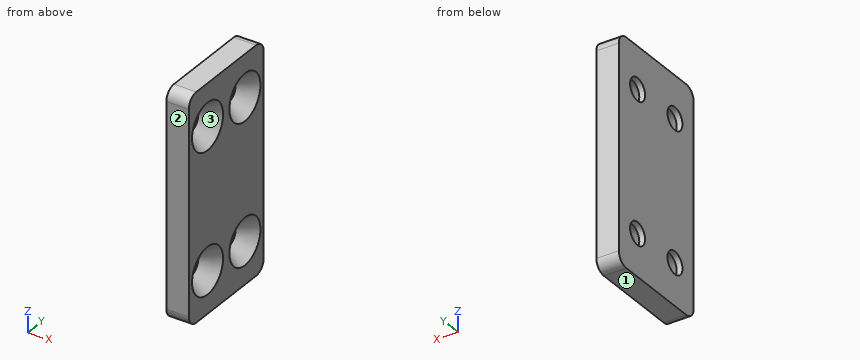
Autodesk Inventor part; units mm, degrees
ref_plane "YZ Plane" through (0, 0, 0) normal (1, 0, 0) x (0, 1, 0)
ref_plane "XZ Plane" through (0, 0, 0) normal (0, 1, 0) x (-1, 0, 0)
ref_plane "XY Plane" through (0, 0, 0) normal (0, 0, 1) x (1, 0, 0)
sketch "Leg_Base_Skt" plane through (0, 0, 0) normal (1, 0, 0) x (0, 1, 0)
  line L0 (-10, -20) -> (10, -20)
  line L1 (10, -20) -> (10, 20)
  line L2 (10, 20) -> (-10, 20)
  line L3 (-10, 20) -> (-10, -20)
  line L4 (-10, -20) -> (10, 20) construction
  line L5 (10, -20) -> (-10, 20) construction
  point P0 (0, 0)
  dimension "d0" = 20
  dimension "d1" = 40
extrude "Leg_Base" add sketch "Leg_Base_Skt" along normal blind 4
sketch "Hole_Base_Skt" plane through (4, 0, 0) normal (1, 0, 0) x (0, 0, -1)
  line L0 (-5, -10) -> (-5, 10) construction
  line L1 (20, 10) -> (-20, 10)
  line L2 (-12.5, 0) -> (-12.5, 10) construction
  line L3 (-12.5, 0) -> (-12.5, -10) construction
  line L4 (-20, -10) -> (20, -10) construction
  line L5 (5, -10) -> (5, 10) construction
  line L6 (20, -10) -> (20, 10) construction
  line L7 (5, 0) -> (20, 0) construction
  line L8 (12.5, 0) -> (12.5, 10) construction
  line L9 (12.5, 0) -> (12.5, -10) construction
  line L10 (-20, 10) -> (-20, -10)
  line L11 (-20, 0) -> (-5, 0) construction
  point P0 (0, 0)
  point P1 (-12.5, -5)
  point P2 (-12.5, 5)
  point P3 (12.5, -5)
  point P4 (12.5, 5)
  dimension "d7" = 15
  dimension "d8" = 15
hole "Hole_Base" at (4, -5, 12.5) at (4, 5, 12.5) at (4, -5, -12.5) at (4, 5, -12.5) direction (-1, 0, 0) diameter 4 end through all countersink diameter 8.3 countersink angle 71.667
fillet "Fillet" radius 2 4 edges at (2, -10, 20) (2, 10, 20) (2, -10, -20) (2, 10, -20)
equation "\"d0\" = block_width"
equation "\"d1\" = ceramic_width + block_height + wood_width"
equation "\"d2\" = screw_head_height + screw_tolerance"
equation "\"d7\" = wood_width"
equation "\"d8\" = block_height"
equation "\"d28\" = screw_body_diam + screw_tolerance"
equation "\"d32\" = screw_head_m"
equation "\"d30\" = screw_head_diam"
equation "\"d33\" = screw_length"
equation "\"d4\" = fillet"
equation "\"tube_diam\" = 31.8"
equation "\"tube_tolerance\" = 0.25"
equation "\"tube_base_height\" = 2"
equation "\"tube_wall_width\" = 3"
equation "\"tube_wall_height\" = 15"
equation "\"screw_wall_width\" = 2"
equation "\"screw_length\" = 12.7"
equation "\"screw_tolerance\" = 1"
equation "\"screw_body_diam\" = 3"
equation "\"screw_head_diam\" = 8.3"
equation "\"screw_head_height\" = 3"
equation "\"screw_spacing\" = 8"
equation "\"block_width\" = 20"
equation "\"block_height\" = 15"
equation "\"ceramic_width\" = 10"
equation "\"wood_width\" = 15"
equation "\"fillet\" = 2"
equation "\"screw_head_m\" = 71.6667deg"
properties part number "Counter_Support_Ceramic_Leg"
Source: CAD feature listing. Evaluate the final solid. Frame: model axes, mm. Face numbers are marked on the shaded views. Give positions to 0.01 mm unless a question says otherwise; leave off trailing zeros. Write each loop counter-clockwise with the first axis right and the second up, starting at its lowest first coordinate (ties: lowest second). Pieces come first, ordered by that corner, then holes. Notation, with made-up numbers: (-35.5, 13) -> (5.5, 13) arc R16 cw to (5.5, 32) -> close; hole circle Ø9 at (47.5, 74). An arc over 180 degrees is marked (long way). Return JSON: item names as keys, results as strings. Group by question number.
1. Section B-B, the plane z = -12.5. Output: boundary loops of the cut face in (x, y).
2. Section C-C, the plane x = 0.4. Output: boundary loops of the cut face in (y, z), then the cut area to 3 significant figures.
3. Mould query, pull axis Z, two halves, no side actions, for the marked faces 1, 2 and 3. Classes: +Z half, -Z half, draft (parallel to the pull), parting line (faces both ways), or undercut.
4. Material intervals for line 1 (Y direction, x = 0.8, z = -12.5); line 2 (Z direction, x = 0.75, y = 5); line 3 (Z direction, x = 1.7, y = 3), sorted ascending. Write a range as from..to.
5. Section A-A, the plane y = 5. Output: boundary loops of the cut face in (x, z).
Determined:
{
 "1": {"outline": "(0, -10) -> (4, -10) -> (4, -9.15) -> (1.02, -7) -> (0, -7) -> close; (0, -3) -> (1.02, -3) -> (4, -0.85) -> (4, 0.85) -> (1.02, 3) -> (0, 3) -> close; (0, 7) -> (1.02, 7) -> (4, 9.15) -> (4, 10) -> (0, 10) -> close"},
 "2": {"outline": "(-10, -18) arc R2 ccw to (-8, -20) -> (8, -20) arc R2 ccw to (10, -18) -> (10, 18) arc R2 ccw to (8, 20) -> (-8, 20) arc R2 ccw to (-10, 18) -> close; hole circle Ø4 at (-5, -12.5); hole circle Ø4 at (-5, 12.5); hole circle Ø4 at (5, -12.5); hole circle Ø4 at (5, 12.5)", "area": "746 mm2"},
 "3": {"face 1": "-Z half", "face 2": "draft", "face 3": "undercut"},
 "4": {"line 1": "y = -10..-7, -3..3, 7..10", "line 2": "z = -20..-14.5, -10.5..10.5, 14.5..20", "line 3": "z = -20..-13.98, -11.02..11.02, 13.98..20"},
 "5": {"outline": "(0, -20) -> (4, -20) -> (4, -16.65) -> (1.02, -14.5) -> (0, -14.5) -> close; (0, -10.5) -> (1.02, -10.5) -> (4, -8.35) -> (4, 8.35) -> (1.02, 10.5) -> (0, 10.5) -> close; (0, 14.5) -> (1.02, 14.5) -> (4, 16.65) -> (4, 20) -> (0, 20) -> close"}
}
